from build123d import *

# Parameters (mm, degrees)
F0_W     = 9.5
F0_H     = 35
F1_DEPTH = 2
F2_R     = 2.45
F3_DEPTH = 8
F4_SIZE  = 1


with BuildPart() as f1:
    # F0 (on Top) → F1 (new body)
    with BuildSketch(Plane.XY):
        with Locations((4.75, 17.5)):
            Rectangle(F0_W, F0_H)
    extrude(amount=F1_DEPTH)

    # F2 (on face) → F3 (join)
    with BuildSketch(Plane.XY.offset(2)):
        with Locations((4.75, 17.5)):
            Circle(F2_R)
    extrude(amount=F3_DEPTH)

    # F4
    f4_edges = [f1.edges().sort_by_distance(p)[0] for p in [
        (2.3, 17.5, 10),
    ]]
    chamfer(f4_edges, length=F4_SIZE)


solid = f1.part
Source: CAD feature listing. Evaluate the final solid. Frame: model axes, mm. Round coordinates to 2 decimals unless told otherwise and drop trailing zeros. Order: outer loops, then holes, each group sorted by start corner. A loop starts at its lowest first (then second) coordinate and runs counter-clockwise, first axis right, second up. Notation, with made-up numbers: (4, 80.5) -> (17, 80.5) arc R20 ccw to (17, 97.5) -> close; hole circle Ø3 at (43.5, -34.75). An arc over 180 degrees is marked (long way). Answer as CSV lines item,"result".
Item 1: Pin query (flat end, axial travel): pin 1 Ø3 at (x, z) = (7.5, 6) entering from -Y; pin 2 Ø5 at (x, y) = (3, 25) entering from +Z. Return the tip coordinate at first contact, or that it passes through.
A:
pin 1,"y = 15.39"
pin 2,"z = 2"
Item 2: Section A-A, the plane y = 17.5. Return loops of the section in (x, z).
A:
outline,"(0, 0) -> (9.5, 0) -> (9.5, 2) -> (7.2, 2) -> (7.2, 9) -> (6.2, 10) -> (3.3, 10) -> (2.3, 9) -> (2.3, 2) -> (0, 2) -> close"
Item 3: Section B-B, the plane x = 4.75. Return loops of the section in (y, z), plus the area to 3 significant figures.
A:
outline,"(0, 0) -> (35, 0) -> (35, 2) -> (19.95, 2) -> (19.95, 9) -> (18.95, 10) -> (16.05, 10) -> (15.05, 9) -> (15.05, 2) -> (0, 2) -> close"
area,"108 mm²"
Item 4: Section C-C, the plane z = 2.75. Return loops of the section in (x, y), plus the area to 3 significant figures.
A:
outline,"circle Ø4.9 at (4.75, 17.5)"
area,"18.9 mm²"
Item 5: Line query: L1, parallel to Z at x = 4.75, y = 21.5; L2, parallel to Y at x = 4.75, z = 3; L3, parallel to X at y = 16, z = 6.5. Output: solid intervals per line, ascending.
A:
L1,"0 to 2"
L2,"15.05 to 19.95"
L3,"2.81 to 6.69"
Item 6: Pull-direction query (Y, two-part tool) for faces 1 (the face through (7.013, 16.562, 5.451)), 2 (the face through (5, 35, 1)), 3 (the face through (5, 18, 10)), 4 (the face through (5, 0, 1)); classes: pulls with the +Y half, pulls with the -Y half, needs draft (parallel to the pull), parting line crosses it, or undercut.
A:
face 1,"parting line crosses it"
face 2,"pulls with the +Y half"
face 3,"needs draft"
face 4,"pulls with the -Y half"
Item 7: Section D-D, the plane x = 8.75. Return loops of the section in (y, z).
A:
outline,"(0, 0) -> (35, 0) -> (35, 2) -> (0, 2) -> close"
